Verification items for the finished model (mm, model axes). Face numbers are marked on the shaded views. Give positions to 0.01 mm unless a question says otherwise; leave off trailing zeros. Order: outer loops, then holes, each group sorted by start corner. A loop starts at its lowest first (then second) coordinate and runs counter-clockwise, first axis right, second up. Notation, with made-up numbers: (43, -16) -> (55, -16) arc R28 cw to (55, 6) -> close; hole circle Ø1 at (74, 85.25). An arc over 180 degrees is marked (long way). One line per question, with ' | ' between items. Start each with the question number.
Q1. Section check D-D on y = -69.5. Record the cut outline in (x, z).
Q2. Section check A-A on z = 0. Record the cut outline in (x, y), plus the area to 3 significant figures.
Q3. Section check C-C on x = 11. Record the cut outline in (y, z), plus the area to 3 significant figures.
Q4. Mould release check, pull along Z, two halves, no side actions. Record for the marked faces 1, 2 and 3: released by +Z, released by -Z, zero draft, split by the parting line, or undercut.
Q5. Go/stop test with flat-tipped pins: pin 1 (5 mm diameter, centred on y = -12, z = -46, fed in from -X); pin 2 (1 mm diameter, centred on x = 23, z = 52.5, fed in from -Y); pin 3 (3 mm diameter, centred on x = 8, y = 62, fed in from +Z); pin 4 (10 mm diameter, centred on x = 12, y = 6, fed in from +Z). Record where each tip stops, or that it passes through.
Q6. Material ranges on probe 1 along Y at (x, z) = (15.5, 0); probe 2 along Y at (x, z) = (21, 0); probe 3 along X at (y, z) = (41, -60.5), recorded low to high. Write a range as [from, to].
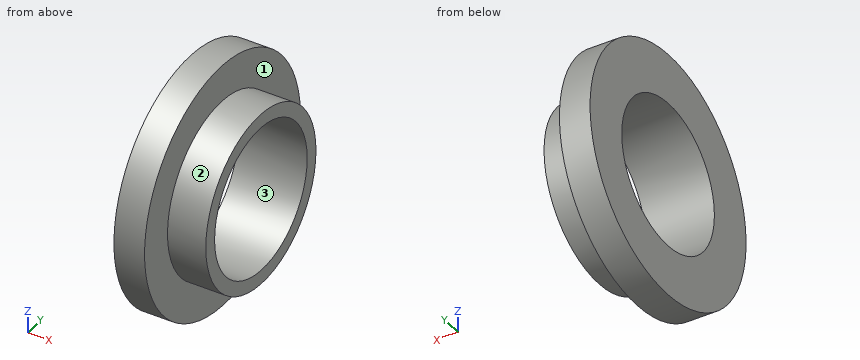
from build123d import *

# Parameters (mm, degrees)
SKETCH_1_R          = 80
EXTRUDE_1_DEPTH     = 45
SKETCH_2_R          = 47.5
CUT_EXTRUDE_1_DEPTH = 122.757956619
SKETCH_3_OUTSIDE_W  = 208.142
SKETCH_3_OUTSIDE_H  = 208.142
SKETCH_3_OUTSIDE_R  = 56.5
CUT_EXTRUDE_2_DEPTH = 25


with BuildPart() as part:
    # 草图1 → 凸台-拉伸1 (new body)
    with BuildSketch(Plane(origin=(0, 0, 0), x_dir=(0, 0, -1), z_dir=(1, 0, 0))):
        with Locations(Location((0, 0, 0), (0, 0, 180))):
            Circle(SKETCH_1_R)
    extrude(amount=EXTRUDE_1_DEPTH)

    # 草图2 → 切除-拉伸1 (cut, through all)
    with BuildSketch(Plane(origin=(45, 0, 0), x_dir=(0, 0, -1), z_dir=(1, 0, 0))):
        Circle(SKETCH_2_R)
    extrude(amount=-CUT_EXTRUDE_1_DEPTH, mode=Mode.SUBTRACT)

    # 草图3 outside → 切除-拉伸2 (cut)
    with BuildSketch(Plane(origin=(45, 0, 0), x_dir=(0, 0, -1), z_dir=(1, 0, 0))):
        Rectangle(SKETCH_3_OUTSIDE_W, SKETCH_3_OUTSIDE_H)
        Circle(SKETCH_3_OUTSIDE_R, mode=Mode.SUBTRACT)
    extrude(amount=-CUT_EXTRUDE_2_DEPTH, mode=Mode.SUBTRACT)


solid = part.part
Filled in:
1) outline: (0, -39.62) -> (20, -39.62) -> (20, 39.62) -> (0, 39.62) -> close
2) outline: (0, -80) -> (20, -80) -> (20, -56.5) -> (45, -56.5) -> (45, -47.5) -> (0, -47.5) -> close; (0, 47.5) -> (45, 47.5) -> (45, 56.5) -> (20, 56.5) -> (20, 80) -> (0, 80) -> close | area: 1,750 mm²
3) outline: circle Ø160 at (0, 0); hole circle Ø95 at (0, 0) | area: 13,000 mm²
4) face 1: zero draft | face 2: split by the parting line | face 3: undercut
5) pin 1: x = 0 | pin 2: y = -22.1 | pin 3: z = 52.34 | pin 4: z = 79.99
6) probe 1: [-80, -47.5], [47.5, 80] | probe 2: [-56.5, -47.5], [47.5, 56.5] | probe 3: [0, 20]
